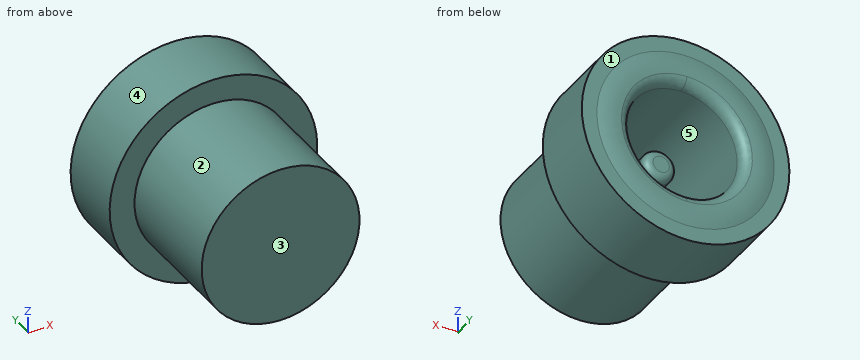
from build123d import *

# Parameters (mm, degrees)
SKETCH1_R           = 4.8
BOSS_EXTRUDE1_DEPTH = 3.2
SKETCH2_R           = 3.65
BOSS_EXTRUDE2_DEPTH = 5.5
SKETCH3_R           = 2.6
CUT_EXTRUDE1_DEPTH  = 8
FILLET1_R           = 0.5
SKETCH5_R           = 0.75
BOSS_EXTRUDE3_DEPTH = 6
FILLET2_R           = 0.375


with BuildPart() as part:
    # Sketch1 → Boss-Extrude1 (new body)
    with BuildSketch(Plane(origin=(0, 0, 0), x_dir=(1, 0, 0), z_dir=(0, 1, 0))):
        with Locations(Location((0, 0, 0), (0, 0, 270))):
            Circle(SKETCH1_R)
    extrude(amount=BOSS_EXTRUDE1_DEPTH)

    # Sketch2 → Boss-Extrude2 (add)
    with BuildSketch(Plane.XZ):
        with Locations(Location((0, 0, 0), (0, 0, 270))):
            Circle(SKETCH2_R)
    extrude(amount=BOSS_EXTRUDE2_DEPTH)

    # Sketch3 → Cut-Extrude1 (cut)
    with BuildSketch(Plane(origin=(0, 3.2, 0), x_dir=(1, 0, 0), z_dir=(0, 1, 0))):
        with Locations(Location((0, 0, 0), (0, 0, 270))):
            Circle(SKETCH3_R)
    extrude(amount=-CUT_EXTRUDE1_DEPTH, mode=Mode.SUBTRACT)

    # Sketch4 → Revolve1 (revolve)
    with BuildSketch(Plane.XY, mode=Mode.PRIVATE) as revolve1_sk:
        with BuildLine():
            Line((-4.1, 3.2), (-2.6, 3.2))
            ThreePointArc((-2.6, 3.2), (-3.35, 3.336000936), (-4.1, 3.2))
        make_face()
    revolve(revolve1_sk.sketch.rotate(Axis((0, 0, 0), (0, 1, 0)), 270), axis=Axis((0, 0, 0), (0, 1, 0)))

    # Fillet1
    fillet1_edges = [part.edges().sort_by_distance(p)[0] for p in [
        (2.6, 3.2, 0),
    ]]
    fillet(fillet1_edges, radius=FILLET1_R)

    # Sketch5 → Boss-Extrude3 (add)
    with BuildSketch(Plane(origin=(0, -4.8, 0), x_dir=(1, 0, 0), z_dir=(0, 1, 0))):
        with Locations(Location((0, 0, 0), (0, 0, 270))):
            Circle(SKETCH5_R)
    extrude(amount=BOSS_EXTRUDE3_DEPTH)

    # Fillet2
    fillet2_edges = [part.edges().sort_by_distance(p)[0] for p in [
        (0, 1.2, -0.75),
    ]]
    fillet(fillet2_edges, radius=FILLET2_R)


solid = part.part
Verification items for the finished model (mm, model axes). Face numbers are marked on the shaded views. A direction names the side the tool comes from. Round coordinates to 2 decimals unless told otherwise and drop trailing zeros. Loops run counter-clockwise (first coordinate to the right, second up) from the corner with the lowest first, then second, coordinate; pieces in that order, holes last. Notation, with made-up numbers: (67.5, 34.5) - (99.5, 34.5) arc R20 ccw to (99.5, 41.5) - close; hole circle Ø5 at (58, 4.5). An arc over 180 degrees is marked (long way). Use a Markdown table: item, result. Add a question column.
1. Section check B-B, the plane y = 2.25. Record the boundary of the cut face in (x, z).
2. Gauge pin test, flat ends, axial feed: pin 1 (1 mm diameter, centred on x = -2.5, z = -3.5, fed in from -Y); pin 2 (1.5 mm diameter, centred on y = -3, z = 1, fed in from +X); pin 3 (1 mm diameter, centred on x = -1, y = 2, fed in from +Z). Record the tip position at first contact, or that the pin passes through.
3. Release check for a two-part mould opening along X. For the marked faces 3, 4 and 5 record: released by +X, released by -X, zero draft, split by the parting line, or undercut.
4. Thickness scan on probe 1 along X at (y, z) = (-1.5, 0); probe 2 along X at (y, z) = (1, 0); probe 3 along Y at (x, z) = (3.25, -2.5). Record the ranges inside material, lowest first. Write a range as [from, to].
5. Section check A-A, the plane y = -3. Record the boundary of the cut face in (x, z).
6. Access from +Z, -Z, +X, -X, +Y, -Y to the whole of each face (thin tool, end or side, straight path). Record for the marked faces 1 and 2.
Checks:
| question | item | result |
|---|---|---|
| 1 | outline | circle Ø9.6 at (0, 0); hole circle Ø5.2 at (0, 0) |
| 2 | pin 1 | stops at y = 0 |
| 2 | pin 2 | stops at x = 3.64 |
| 2 | pin 3 | stops at z = 4.77 |
| 3 | face 3 | zero draft |
| 3 | face 4 | split by the parting line |
| 3 | face 5 | undercut |
| 4 | probe 1 | x = [-3.65, -2.6], [-0.75, 0.75], [2.6, 3.65] |
| 4 | probe 2 | x = [-4.8, -2.6], [-0.71, 0.71], [2.6, 4.8] |
| 4 | probe 3 | y = [0, 3.2] |
| 5 | outline | circle Ø7.3 at (0, 0); circle Ø1.5 at (0, 0); hole circle Ø5.2 at (0, 0) |
| 6 | face 1 | +Y |
| 6 | face 2 | -Y |
